Autodesk Inventor part; units mm, degrees
ref_plane "Work Plane1" through (0, 0, 39) normal (0, 0, 1) x (1, 0, 0)
ref_plane "YZ Plane" through (0, 0, 0) normal (1, 0, 0) x (0, 1, 0)
ref_plane "XZ Plane" through (0, 0, 0) normal (0, 1, 0) x (-1, 0, 0)
sketch "Sketch1" plane through (0, 0, 0) normal (0, 0, 1) x (1, 0, 0)
  circle A0 centre (0, 0) radius 11
  dimension "d0" = 22
extrude "Extrusion1" add sketch "Sketch1" along normal blind 45
ref_plane "Work Plane1" through (0, 0, 39) normal (0, 0, 1) x (1, 0, 0)
sketch "Sketch2" plane through (0, 0, 39) normal (0, 0, 1) x (1, 0, 0)
  circle A0 centre (0, 0) radius 22.25
  circle A1 centre (0, 17.5) radius 2.5
  circle A2 centre (-15.1554, -8.75) radius 2.5
  circle A3 centre (15.1554, -8.75) radius 2.5
  dimension "d4" = 44.5
  dimension "d5" = 5
  dimension "d6" = 17.5
  dimension "d9" = 360
extrude "Extrusion2" add sketch "Sketch2" against normal blind 2.3
sketch "Sketch3" plane through (0, 0, 45) normal (0, 0, 1) x (1, 0, 0)
  circle A0 centre (0, 0) radius 3.5
  dimension "d13" = 7
extrude "Extrusion3" add sketch "Sketch3" along normal blind 7
properties part number "Slip Ring" material "ABS Plastic"
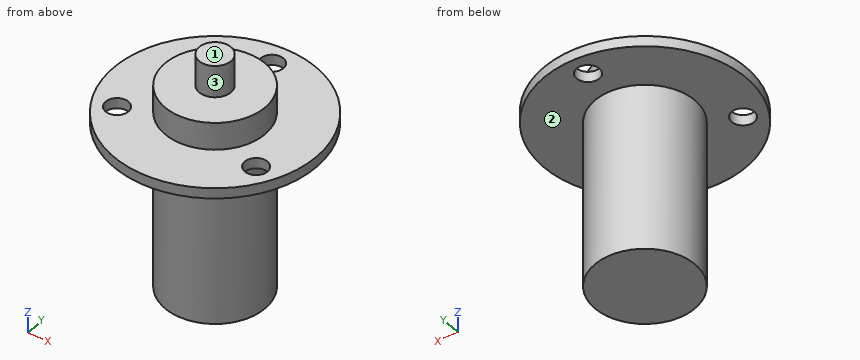
Here's how the part is built. I have some questions about the finished solid (model axes, mm). Face numbers are marked on the shaded views. A direction names the side the tool comes from. Round coordinates to 2 decimals unless told otherwise and drop trailing zeros. Order: outer loops, then holes, each group sorted by start corner. A loop starts at its lowest first (then second) coordinate and runs counter-clockwise, first axis right, second up. Notation, with made-up numbers: M 5,-21.75 L 31,-21.75 A26 cw 31,10.25 Z; hole C 6,25.25 d1. An arc over 180 degrees is marked long. One line per question, with ' | ' between items.
1) I'm going to push flat-ended pins straight in: pin 1 Ø10 at (y, z) = (-9.5, 23.5) entering from -X; pin 2 Ø2 at (y, z) = (8, 34.5) entering from -X; pin 3 Ø12 at (y, z) = (-15.5, 29.5) entering from +X. Where does each tip first touch, or does it pass through?
Checked values:
pin 1: stops at x = -10.04 | pin 2: stops at x = -8.49 | pin 3: stops at x = 5.55
2) Imagine slicing it at A-A, the plane x = -17. Write out the boundary of the cut face in (y, z).
Checked values:
outline: M -14.35,36.7 L -10.44,36.7 L -10.44,39 L -14.35,39 Z; M -7.06,36.7 L 14.35,36.7 L 14.35,39 L -7.06,39 Z
3) Imagine slicing it at B-B, the plane y = 0. Write out the boundary of the cut face in (x, z).
Checked values:
outline: M -22.25,36.7 L -11,36.7 L -11,0 L 11,0 L 11,36.7 L 22.25,36.7 L 22.25,39 L 11,39 L 11,45 L 3.5,45 L 3.5,52 L -3.5,52 L -3.5,45 L -11,45 L -11,39 L -22.25,39 Z
4) On a 3-axis mill with a long thin cutter (end or side, diameter ignored), from which of +Z, -Z, +X, -X, +Y, -Y can I reach the whole of each face in a straight line? I mean the marked faces 1, 2 and 3. Say none if no direction works.
Checked values:
face 1: +Z, +X, -X, +Y, -Y | face 2: -Z | face 3: +Z
5) Imagine slicing it at C-C, the plane y = 17.5. Write out the boundary of the cut face in (x, z), plus the area to 3 significant figures.
Checked values:
outline: M -13.74,36.7 L -2.5,36.7 L -2.5,39 L -13.74,39 Z; M 2.5,36.7 L 13.74,36.7 L 13.74,39 L 2.5,39 Z | area: 51.7 mm²
6) Imagine slicing it at D-D, the plane x = -6. Write out the boundary of the cut face in (y, z).
Checked values:
outline: M -21.43,36.7 L -9.22,36.7 L -9.22,0 L 9.22,0 L 9.22,36.7 L 21.43,36.7 L 21.43,39 L 9.22,39 L 9.22,45 L -9.22,45 L -9.22,39 L -21.43,39 Z
7) I need wall thicknesses on line 1 (Y direction, x = 0, z = 38.35); line 2 (Z direction, x = -6, y = 17.5); line 3 (X direction, y = 17, z = 37). Which ranges of each line are inside material? Lowest first, please.
Checked values:
line 1: y = -22.25 to 15, 20 to 22.25 | line 2: z = 36.7 to 39 | line 3: x = -14.35 to -2.45, 2.45 to 14.35
